```python
from build123d import *

# Parameters (mm, degrees)
BASE_FLANGE1_DEPTH = 1
EDGE_FLANGE1_DEPTH = 39
FILLET1_R          = 3
SKETCH12_R         = 15.241955925
SKETCH12_R_2       = 0.968487673
CUT_EXTRUDE1_DEPTH = 1
SKETCH13_R         = 1.066611422
CUT_EXTRUDE2_DEPTH = 1


# Sheet-metal steps are written as plain solids
with BuildPart() as part:
    # Sketch2 → Base-Flange1 (new body)
    with BuildSketch(Plane.XY):
        with BuildLine():
            Line((0, 0), (39, 0))
            Line((39, 0), (39, 33))
            ThreePointArc((39, 33), (37.242640687, 37.242640687), (33, 39))
            Line((33, 39), (6, 39))
            ThreePointArc((6, 39), (1.757359313, 37.242640687), (0, 33))
            Line((0, 33), (0, 0))
        make_face()
    extrude(amount=-BASE_FLANGE1_DEPTH)

    # Edge-Flange1 section (across the edge) → Edge-Flange1 (add)
    with BuildSketch(Plane(origin=(39, -0.7366, -1), x_dir=(0, 1, 0), z_dir=(-1, 0, 0))):
        with BuildLine():
            Line((-1, 0.7366), (-1, 21))
            Line((-1, 21), (0, 21))
            Line((0, 21), (0, 0.7366))
            ThreePointArc((0, 0.7366), (0.215745145, 0.215745145), (0.7366, 0))
            Line((0.7366, 0), (0.7366, -1))
            ThreePointArc((0.7366, -1), (-0.491361636, -0.491361636), (-1, 0.7366))
        make_face()
    extrude(amount=EDGE_FLANGE1_DEPTH)

    # Fillet1
    fillet1_edges = [part.edges().sort_by_distance(p)[0] for p in [
        (39, -1.2366, -22),
        (0, -1.2366, -22),
    ]]
    fillet(fillet1_edges, radius=FILLET1_R)

    # Sketch12 → Cut-Extrude1 (cut)
    with BuildSketch(Plane(origin=(0, 0, -1), x_dir=(-1, 0, 0), z_dir=(0, 0, -1))):
        with Locations((-19.5, 19.5)):
            Circle(SKETCH12_R)
        with Locations((-19.5, 36.110428889)):
            Circle(SKETCH12_R_2)
        with Locations((-27.805214445, 33.885053386)):
            Circle(SKETCH12_R_2)
        with Locations((-33.885053386, 27.805214445)):
            Circle(SKETCH12_R_2)
        with Locations((-36.110428889, 19.5)):
            Circle(SKETCH12_R_2)
        with Locations((-33.885053386, 11.194785555)):
            Circle(SKETCH12_R_2)
        with Locations((-27.805214445, 5.114946614)):
            Circle(SKETCH12_R_2)
        with Locations((-19.5, 2.889571111)):
            Circle(SKETCH12_R_2)
        with Locations((-11.194785555, 5.114946614)):
            Circle(SKETCH12_R_2)
        with Locations((-5.114946614, 11.194785555)):
            Circle(SKETCH12_R_2)
        with Locations((-2.889571111, 19.5)):
            Circle(SKETCH12_R_2)
        with Locations((-5.114946614, 27.805214445)):
            Circle(SKETCH12_R_2)
        with Locations((-11.194785555, 33.885053386)):
            Circle(SKETCH12_R_2)
    extrude(amount=-CUT_EXTRUDE1_DEPTH, mode=Mode.SUBTRACT)

    # Sketch13 → Cut-Extrude2 (cut)
    with BuildSketch(Plane(origin=(0, -0.7366, 0), x_dir=(1, 0, 0), z_dir=(0, 1, 0))):
        with Locations(Location((3.175481607, 18.89157203, 0), (0, 0, 270))):
            Circle(SKETCH13_R)
        with Locations(Location((3.175481607, 11.89157203, 0), (0, 0, 270))):
            Circle(SKETCH13_R)
        with Locations(Location((3.175481607, 4.89157203, 0), (0, 0, 270))):
            Circle(SKETCH13_R)
        with Locations(Location((35.824518393, 4.89157203, 0), (0, 0, 90))):
            Circle(SKETCH13_R)
        with Locations(Location((35.824518393, 11.89157203, 0), (0, 0, 90))):
            Circle(SKETCH13_R)
        with Locations(Location((35.824518393, 18.89157203, 0), (0, 0, 90))):
            Circle(SKETCH13_R)
    extrude(amount=-CUT_EXTRUDE2_DEPTH, mode=Mode.SUBTRACT)


solid = part.part
```
Could you check a few things on this model? Use its own coordinates, in mm. Round coordinates to 2 decimals unless told otherwise and drop trailing zeros. Write each loop counter-clockwise with the first axis right and the second up, starting at its lowest first coordinate (ties: lowest second). Pieces come first, ordered by that corner, then holes. Notation, with made-up numbers: M 46.25,80.25 L 91.25,80.25 A18 cw 91.25,105.25 Z; hole C 45,41 d2. An arc over 180 degrees is marked long. Answer in a Markdown table with one row per item. Add a question column.
Q1. If we mould it in two halves opening along X, with no side actions, what happens to faces 1 (the cylindrical face through (19.773, -1.214, -0.495)), 2 (the cylindrical face through (5.32, 10.25, -0.51)), 3 (the cylindrical face through (19.053, 35.251, -0.507)), 4 (the flat face through (0, 8, -0.4))? For each: +X half, -X half, draft (parallel to the pull), parting line (faces both ways), or undercut.
Q2. Will these pins go through, and if not, where does the flat tip stop? pin 1 Ø4 at (x, z) = (19.5, -5) entering from +Y; pin 2 Ø10 at (x, y) = (30.5, 5) entering from -Z.
Q3. Imagine slicing it at A-A (x = 19.5). Please give me the cut outline in (y, z), then the cut area to 3 significant figures.
Q4. Imagine slicing it at B-B (y = 19.5). Please give me the cut outline in (x, z), then the cut area to 3 significant figures.
Q5. If I drill on line 1 (Y direction, x = 8, z = -9.75); line 2 (Z direction, x = 36.5, y = 32.5), over which ranges is the centre line in solid material (lowest first)? Write a range as from..to.
Q6. Imagine slicing it at D-D (x = 26). Please give me the cut outline in (y, z).
Q7. Imagine slicing it at C-C (y = 26). Please give me the cut outline in (x, z).
Values:
| question | item | result |
|---|---|---|
| 1 | face 1 | draft |
| 1 | face 2 | undercut |
| 1 | face 3 | undercut |
| 1 | face 4 | -X half |
| 2 | pin 1 | y = -0.74 |
| 2 | pin 2 | z = -1 |
| 3 | outline | M -1.74,-22 L -0.74,-22 L -0.74,-1.74 A0.74 cw 0,-1 L 1.92,-1 L 1.92,0 L 0,0 A1.74 ccw -1.74,-1.74 Z; M 3.86,-1 L 4.26,-1 L 4.26,0 L 3.86,0 Z; M 34.74,-1 L 35.14,-1 L 35.14,0 L 34.74,0 Z; M 37.08,-1 L 39,-1 L 39,0 L 37.08,0 Z |
| 3 | area | 26.8 mm^2 |
| 4 | outline | M 0,-1 L 1.92,-1 L 1.92,0 L 0,0 Z; M 3.86,-1 L 4.26,-1 L 4.26,0 L 3.86,0 Z; M 34.74,-1 L 35.14,-1 L 35.14,0 L 34.74,0 Z; M 37.08,-1 L 39,-1 L 39,0 L 37.08,0 Z |
| 4 | area | 4.64 mm^2 |
| 5 | line 1 | -1.74..-0.74 |
| 5 | line 2 | -1..0 |
| 6 | outline | M -1.74,-22 L -0.74,-22 L -0.74,-1.74 A0.74 cw 0,-1 L 5.71,-1 L 5.71,0 L 0,0 A1.74 ccw -1.74,-1.74 Z; M 33.29,-1 L 39,-1 L 39,0 L 33.29,0 Z |
| 7 | outline | M 0,-1 L 5.71,-1 L 5.71,0 L 0,0 Z; M 33.29,-1 L 39,-1 L 39,0 L 33.29,0 Z |
